Build history of the part. All positions in model axes, mm. Coordinates: 2 decimals unless noted, no trailing zeros. Loops run counter-clockwise (first coordinate to the right, second up) from the corner with the lowest first, then second, coordinate; pieces in that order, holes last.
Item 1: Cut at A-A (y = 2.75). List the corners of the cut face in (x, z).
Item 2: Cut at D-D (y = 8.75). List the corners of the cut face in (x, z), and give its area (3 significant figures).
Item 3: Flat gauge pins, fed straight in: pin 1 (8 mm diameter, centred on x = 30, y = 9.5, fed in from -Z); pin 2 (12 mm diameter, centred on x = 42, y = -2.5, fed in from +Z). Where does each tip first touch, or does it go through?
Item 4: Cut at B-B (x = 32). List the corners of the cut face in (y, z).
Item 5: Cut at C-C (x = 2). List the corners of the cut face in (y, z).
Item 6: Drill centre lines: line 1 along Z through (x, y) = (34, -7.5); line 2 along X through (y, z) = (11.25, -2.3). Where is each one in solid material? Low to high.
from build123d import *

# Parameters (mm, degrees)
F0_W     = 14.2
F0_H     = 13
F1_DEPTH = 0.15
F2_W     = 0.15
F2_H     = 7
F3_DEPTH = 5
F4_R     = 0.5
F6_DEPTH = 25


with BuildPart() as f1:
    # F0 (on Top) → F1 (new body)
    with BuildSketch(Plane.XY):
        with BuildLine():
            Line((-13.1, 10.5), (-13.1, 13.5))
            Line((-13.1, 13.5), (-22.1, 13.5))
            Line((-22.1, 13.5), (-22.1, 6.5))
            Line((-22.1, 6.5), (-13.1, 6.5))
            Line((-13.1, 6.5), (-13.1, 9.5))
            Line((-13.1, 9.5), (-14.7, 9.5))
            ThreePointArc((-14.7, 9.5), (-14.9828427125, 9.6171572875), (-15.1, 9.9))
            Line((-15.1, 9.9), (-15.1, 10.1))
            ThreePointArc((-15.1, 10.1), (-14.9828427125, 10.3828427125), (-14.7, 10.5))
            Line((-14.7, 10.5), (-13.1, 10.5))
        make_face()
        with BuildLine():
            Line((53.5, 13.5), (33.3, 13.5))
            Line((33.3, 13.5), (33.3, 10.5))
            Line((33.3, 10.5), (34.9, 10.5))
            ThreePointArc((34.9, 10.5), (35.1828427125, 10.3828427125), (35.3, 10.1))
            Line((35.3, 10.1), (35.3, 9.9))
            ThreePointArc((35.3, 9.9), (35.1828427125, 9.6171572875), (34.9, 9.5))
            Line((34.9, 9.5), (33.3, 9.5))
            Line((33.3, 9.5), (33.3, 6.5))
            Line((33.3, 6.5), (47.5, 6.5))
            Line((47.5, 6.5), (47.5, -6.5))
            Line((47.5, -6.5), (33.3, -6.5))
            Line((33.3, -6.5), (33.3, -9.5))
            Line((33.3, -9.5), (34.9, -9.5))
            ThreePointArc((34.9, -9.5), (35.1828427125, -9.6171572875), (35.3, -9.9))
            Line((35.3, -9.9), (35.3, -10.1))
            ThreePointArc((35.3, -10.1), (35.1828427125, -10.3828427125), (34.9, -10.5))
            Line((34.9, -10.5), (33.3, -10.5))
            Line((33.3, -10.5), (33.3, -13.5))
            Line((33.3, -13.5), (53.5, -13.5))
            Line((53.5, -13.5), (53.5, -10.5))
            Line((53.5, -10.5), (45.9, -10.5))
            ThreePointArc((45.9, -10.5), (45.6171572875, -10.3828427125), (45.5, -10.1))
            Line((45.5, -10.1), (45.5, -9.9))
            ThreePointArc((45.5, -9.9), (45.6171572875, -9.6171572875), (45.9, -9.5))
            Line((45.9, -9.5), (53.5, -9.5))
            Line((53.5, -9.5), (53.5, 0))
            Line((53.5, 0), (53.5, 9.5))
            Line((53.5, 9.5), (45.9, 9.5))
            ThreePointArc((45.9, 9.5), (45.6171572875, 9.6171572875), (45.5, 9.9))
            Line((45.5, 9.9), (45.5, 10.1))
            ThreePointArc((45.5, 10.1), (45.6171572875, 10.3828427125), (45.9, 10.5))
            Line((45.9, 10.5), (53.5, 10.5))
            Line((53.5, 10.5), (53.5, 13.5))
        make_face()
        with BuildLine():
            Line((13.1, 10.5), (13.1, 13.5))
            Line((13.1, 13.5), (-7.1, 13.5))
            Line((-7.1, 13.5), (-13.1, 13.5))
            Line((-13.1, 13.5), (-13.1, 10.5))
            Line((-13.1, 10.5), (-5.5, 10.5))
            ThreePointArc((-5.5, 10.5), (-5.2171572875, 10.3828427125), (-5.1, 10.1))
            Line((-5.1, 10.1), (-5.1, 9.9))
            ThreePointArc((-5.1, 9.9), (-5.2171572875, 9.6171572875), (-5.5, 9.5))
            Line((-5.5, 9.5), (-13.1, 9.5))
            Line((-13.1, 9.5), (-13.1, 6.5))
            Line((-13.1, 6.5), (-13.1, 0))
            Line((-13.1, 0), (-13.1, -6.5))
            Line((-13.1, -6.5), (-13.1, -9.5))
            Line((-13.1, -9.5), (-5.5, -9.5))
            ThreePointArc((-5.5, -9.5), (-5.2171572875, -9.6171572875), (-5.1, -9.9))
            Line((-5.1, -9.9), (-5.1, -10.1))
            ThreePointArc((-5.1, -10.1), (-5.2171572875, -10.3828427125), (-5.5, -10.5))
            Line((-5.5, -10.5), (-13.1, -10.5))
            Line((-13.1, -10.5), (-13.1, -13.5))
            Line((-13.1, -13.5), (-7.1, -13.5))
            Line((-7.1, -13.5), (13.1, -13.5))
            Line((13.1, -13.5), (13.1, -10.5))
            Line((13.1, -10.5), (5.5, -10.5))
            ThreePointArc((5.5, -10.5), (5.2171572875, -10.3828427125), (5.1, -10.1))
            Line((5.1, -10.1), (5.1, -9.9))
            ThreePointArc((5.1, -9.9), (5.2171572875, -9.6171572875), (5.5, -9.5))
            Line((5.5, -9.5), (13.1, -9.5))
            Line((13.1, -9.5), (13.1, -6.5))
            Line((13.1, -6.5), (13.1, 0))
            Line((13.1, 0), (13.1, 6.5))
            Line((13.1, 6.5), (13.1, 9.5))
            Line((13.1, 9.5), (5.5, 9.5))
            ThreePointArc((5.5, 9.5), (5.2171572875, 9.6171572875), (5.1, 9.9))
            Line((5.1, 9.9), (5.1, 10.1))
            ThreePointArc((5.1, 10.1), (5.2171572875, 10.3828427125), (5.5, 10.5))
            Line((5.5, 10.5), (13.1, 10.5))
        make_face()
        Rectangle(F0_W, F0_H, mode=Mode.SUBTRACT)
        with BuildLine():
            Line((33.3, 13.5), (13.1, 13.5))
            Line((13.1, 13.5), (13.1, 10.5))
            Line((13.1, 10.5), (14.7, 10.5))
            ThreePointArc((14.7, 10.5), (14.9828427125, 10.3828427125), (15.1, 10.1))
            Line((15.1, 10.1), (15.1, 9.9))
            ThreePointArc((15.1, 9.9), (14.9828427125, 9.6171572875), (14.7, 9.5))
            Line((14.7, 9.5), (13.1, 9.5))
            Line((13.1, 9.5), (13.1, 6.5))
            Line((13.1, 6.5), (27.3, 6.5))
            Line((27.3, 6.5), (27.3, -6.5))
            Line((27.3, -6.5), (13.1, -6.5))
            Line((13.1, -6.5), (13.1, -9.5))
            Line((13.1, -9.5), (14.7, -9.5))
            ThreePointArc((14.7, -9.5), (14.9828427125, -9.6171572875), (15.1, -9.9))
            Line((15.1, -9.9), (15.1, -10.1))
            ThreePointArc((15.1, -10.1), (14.9828427125, -10.3828427125), (14.7, -10.5))
            Line((14.7, -10.5), (13.1, -10.5))
            Line((13.1, -10.5), (13.1, -13.5))
            Line((13.1, -13.5), (33.3, -13.5))
            Line((33.3, -13.5), (33.3, -10.5))
            Line((33.3, -10.5), (25.7, -10.5))
            ThreePointArc((25.7, -10.5), (25.4171572875, -10.3828427125), (25.3, -10.1))
            Line((25.3, -10.1), (25.3, -9.9))
            ThreePointArc((25.3, -9.9), (25.4171572875, -9.6171572875), (25.7, -9.5))
            Line((25.7, -9.5), (33.3, -9.5))
            Line((33.3, -9.5), (33.3, -6.5))
            Line((33.3, -6.5), (33.3, 0))
            Line((33.3, 0), (33.3, 6.5))
            Line((33.3, 6.5), (33.3, 9.5))
            Line((33.3, 9.5), (25.7, 9.5))
            ThreePointArc((25.7, 9.5), (25.4171572875, 9.6171572875), (25.3, 9.9))
            Line((25.3, 9.9), (25.3, 10.1))
            ThreePointArc((25.3, 10.1), (25.4171572875, 10.3828427125), (25.7, 10.5))
            Line((25.7, 10.5), (33.3, 10.5))
            Line((33.3, 10.5), (33.3, 13.5))
        make_face()
    extrude(amount=F1_DEPTH)

    # F2 (on face) → F3 (join)
    with BuildSketch(Plane(origin=(0, 0, 0), x_dir=(1, 0, 0), z_dir=(0, 0, -1))):
        with Locations((-22.025, -10)):
            Rectangle(F2_W, F2_H)
    extrude(amount=F3_DEPTH)

    # F4
    f4_edges = [f1.edges().sort_by_distance(p)[0] for p in [
        (-21.95, 10, 0),
        (-22.1, 10, 0.15),
    ]]
    fillet(f4_edges, radius=F4_R)

    # F5 (on face) → F6 (cut)
    with BuildSketch(Plane(origin=(-22.1, 0, 0), x_dir=(0, -1, 0), z_dir=(-1, 0, 0))):
        with BuildLine():
            Line((-9.9, -3.35), (-10, -3.35))
            Line((-10, -3.35), (-10.1, -3.35))
            ThreePointArc((-10.1, -3.35), (-10.3828427125, -3.4671572875), (-10.5, -3.75))
            Line((-10.5, -3.75), (-10.5, -5))
            Line((-10.5, -5), (-9.5, -5))
            Line((-9.5, -5), (-9.5, -3.75))
            ThreePointArc((-9.5, -3.75), (-9.6171572875, -3.4671572875), (-9.9, -3.35))
        make_face()
    extrude(amount=-F6_DEPTH, mode=Mode.SUBTRACT)


solid = f1.part
Filled sheet:
1. outline: (-13.1, 0) - (-7.1, 0) - (-7.1, 0.15) - (-13.1, 0.15) - close; (7.1, 0) - (13.1, 0) - (13.1, 0.15) - (7.1, 0.15) - close; (27.3, 0) - (33.3, 0) - (33.3, 0.15) - (27.3, 0.15) - close; (47.5, 0) - (53.5, 0) - (53.5, 0.15) - (47.5, 0.15) - close
2. outline: (-22.1, -5) - (-21.95, -5) - (-21.95, -0.5) arc R0.5 cw to (-21.45, 0) - (53.5, 0) - (53.5, 0.15) - (-21.6, 0.15) arc R0.5 ccw to (-22.1, -0.35) - close
2. area: 12.1 mm2
3. pin 1: stops at z = 0
3. pin 2: stops at z = 0.15
4. outline: (-13.5, 0) - (-10.5, 0) - (-10.5, 0.15) - (-13.5, 0.15) - close; (-9.5, 0) - (9.5, 0) - (9.5, 0.15) - (-9.5, 0.15) - close; (10.5, 0) - (13.5, 0) - (13.5, 0.15) - (10.5, 0.15) - close
5. outline: (-13.5, 0) - (-6.5, 0) - (-6.5, 0.15) - (-13.5, 0.15) - close; (6.5, 0) - (13.5, 0) - (13.5, 0.15) - (6.5, 0.15) - close
6. line 1: z = 0 to 0.15
6. line 2: x = -22.1 to -21.95
